```python
from build123d import *

# Parameters (mm, degrees)
F0_R     = 7.5
F1_DEPTH = 20
F2_R     = 5
F3_DEPTH = 16
F4_SIZE  = 2
F5_R     = 1
F6_R     = 3


with BuildPart() as f1:
    # F0 (on Top) → F1 (new body)
    with BuildSketch(Plane.XY):
        Circle(F0_R)
    extrude(amount=F1_DEPTH)

    # F2 (on face) → F3 (cut)
    with BuildSketch(Plane.XY.offset(20)):
        Circle(F2_R)
    extrude(amount=-F3_DEPTH, mode=Mode.SUBTRACT)

    # F4
    f4_edges = [f1.edges().sort_by_distance(p)[0] for p in [
        (-7.5, 0, 0),
    ]]
    chamfer(f4_edges, length=F4_SIZE)

    # F5
    f5_edges = [f1.edges().sort_by_distance(p)[0] for p in [
        (-7.5, 0, 20),
        (-5, 0, 20),
    ]]
    fillet(f5_edges, radius=F5_R)

    # F6
    f6_edges = [f1.edges().sort_by_distance(p)[0] for p in [
        (-5, 0, 4),
    ]]
    fillet(f6_edges, radius=F6_R)


solid = f1.part
```
The listing builds one solid part. Answer for the finished solid, in the listing's coordinates (mm). A direction names the side the tool comes from. Round coordinates to 2 decimals unless told otherwise and drop trailing zeros. Loops run counter-clockwise (first coordinate to the right, second up) from the corner with the lowest first, then second, coordinate; pieces in that order, holes last.
Q1. Which of the six approach directions +Z, -Z, +X, -X, +Y, -Y give full straight-line access (tool end or side, diameter ignored) to faces 1 (the face through (0, 0, 0)), 2 (the face through (0, 0, 4))?
Q2. Given pin 1 Ø1 at (y, z) = (3, 10) entering from +X; pin 2 Ø1 at (x, z) = (5.5, 8.5) entering from -Y; pin 3 Ø2 at (x, y) = (-0.5, -0.5) entering from +Z, each flat-ended and moving along its own axis, determine where each tip first touches the part or whether it passes through.
Q3. For a pull along X with two mould halves and no side action, classify faces 3 (the face through (-7.493, 0.33, 10.381)), 4 (the face through (2, -6, 20)), 5 (the face through (-1.08, -4.88, 13.08)) as released by +X, released by -X, zero draft, split by the parting line, or undercut.
Q4. Section A-A, the plane z = 10.5 is taken. Determine the outline of the cut face in (x, y).
Q5. Find the intervals of material crossed by line 1 (Y direction, x = 0, z = 14); line 2 (Y direction, x = 2.25, z = 8.75); line 3 (X direction, y = -1, z = 5.5), in increasing order.
Completed:
1. face 1: -Z, +X, -X, +Y, -Y
1. face 2: +Z
2. pin 1: stops at x = 7.07
2. pin 2: stops at y = -5.59
2. pin 3: stops at z = 4
3. face 3: split by the parting line
3. face 4: zero draft
3. face 5: undercut
4. outline: circle Ø15 at (0, 0); hole circle Ø10 at (0, 0)
5. line 1: y = -7.5 to -5, 5 to 7.5
5. line 2: y = -7.15 to -4.47, 4.47 to 7.15
5. line 3: x = -7.43 to -4.49, 4.49 to 7.43
